Work out the finished part from the listing and answer in its coordinate system (mm). A direction names the side the tool comes from. Give positions to 0.01 mm unless a question says otherwise; leave off trailing zeros. Order: outer loops, then holes, each group sorted by start corner. A loop starts at its lowest first (then second) coordinate and runs counter-clockwise, first axis right, second up.
```python
from build123d import *

# Parameters (mm, degrees)
BOSS_EXTRUDE1_DEPTH = 10
SKETCH2_W           = 20
SKETCH2_H           = 14
BOSS_EXTRUDE2_DEPTH = 20
SKETCH3_W           = 20
SKETCH3_H           = 5
BOSS_EXTRUDE3_DEPTH = 20
SKETCH4_R           = 1.75
CUT_EXTRUDE1_DEPTH  = 84.402637848
CIRPATTERN1_COUNT   = 3
SKETCH5_R           = 2.5
CUT_EXTRUDE2_DEPTH  = 117.266161556
SKETCH8_W           = 20
SKETCH8_H           = 14
BOSS_EXTRUDE7_DEPTH = 5
SKETCH11_W          = 52
SKETCH11_H          = 52
BOSS_EXTRUDE8_DEPTH = 10
CUT_EXTRUDE3_DEPTH  = 7


with BuildPart() as part:
    # Sketch1 → Boss-Extrude1 (new body)
    with BuildSketch(Plane(origin=(0, 0, 0), x_dir=(1, 0, 0), z_dir=(0, 1, 0))):
        Polygon((0, 0), (-10, 5.773502692), (-10, 80), (10, 80), (10, 5.773502692), align=None)
    boss_extrude1 = extrude(amount=BOSS_EXTRUDE1_DEPTH)

    # Sketch2 → Boss-Extrude2 (add)
    with BuildSketch(Plane(origin=(0, 10, 0), x_dir=(1, 0, 0), z_dir=(0, 1, 0))):
        with Locations((0, 73)):
            Rectangle(SKETCH2_W, SKETCH2_H)
    boss_extrude2 = extrude(amount=BOSS_EXTRUDE2_DEPTH)

    # Sketch3 → Boss-Extrude3 (add)
    with BuildSketch(Plane(origin=(0, 30, 0), x_dir=(1, 0, 0), z_dir=(0, 1, 0))):
        with Locations((0, 77.5)):
            Rectangle(SKETCH3_W, SKETCH3_H)
        with Locations((0, 68.5)):
            Rectangle(SKETCH3_W, SKETCH3_H)
    boss_extrude3 = extrude(amount=BOSS_EXTRUDE3_DEPTH)

    # Sketch4 → Cut-Extrude1 (cut, symmetric)
    with BuildSketch(Plane.XY.offset(-66)):
        with Locations((0, 47)):
            Circle(SKETCH4_R)
    cut_extrude1 = extrude(amount=CUT_EXTRUDE1_DEPTH, both=True, mode=Mode.SUBTRACT)

    # CirPattern1: Boss-Extrude1, Boss-Extrude2, Boss-Extrude3, Cut-Extrude1 ×3 about axis
    cirpattern1_axis = Axis((0, 0, 0), (0, 1, 0))
    add([boss_extrude1.rotate(cirpattern1_axis, i * 360 / CIRPATTERN1_COUNT) for i in range(1, CIRPATTERN1_COUNT)])
    add([boss_extrude2.rotate(cirpattern1_axis, i * 360 / CIRPATTERN1_COUNT) for i in range(1, CIRPATTERN1_COUNT)])
    add([boss_extrude3.rotate(cirpattern1_axis, i * 360 / CIRPATTERN1_COUNT) for i in range(1, CIRPATTERN1_COUNT)])
    add([cut_extrude1.rotate(cirpattern1_axis, i * 360 / CIRPATTERN1_COUNT) for i in range(1, CIRPATTERN1_COUNT)], mode=Mode.SUBTRACT)

    # Sketch5 → Cut-Extrude2 (cut, through all)
    with BuildSketch(Plane(origin=(0, 10, 0), x_dir=(1, 0, 0), z_dir=(0, 1, 0))):
        with Locations(Location((0, 0, 0), (0, 0, 270))):
            Circle(SKETCH5_R)
    extrude(amount=-CUT_EXTRUDE2_DEPTH, mode=Mode.SUBTRACT)

    # Sketch8 → Boss-Extrude7 (add)
    with BuildSketch(Plane(origin=(0, 0, 0), x_dir=(1, 0, 0), z_dir=(0, 1, 0))):
        with Locations((0, 87)):
            Rectangle(SKETCH8_W, SKETCH8_H)
    extrude(amount=BOSS_EXTRUDE7_DEPTH)

    # Sketch11 → Boss-Extrude8 (add)
    with BuildSketch(Plane(origin=(0, 0, 0), x_dir=(1, 0, 0), z_dir=(0, 1, 0))):
        with Locations((0, 120)):
            Rectangle(SKETCH11_W, SKETCH11_H)
    extrude(amount=BOSS_EXTRUDE8_DEPTH)

    # Sketch12 → Cut-Extrude3 (cut)
    with BuildSketch(Plane(origin=(0, 10, 0), x_dir=(1, 0, 0), z_dir=(0, 1, 0))):
        Polygon((-21.1, 141.1), (-10.1, 141.1), (-10.1, 146), (10.1, 146), (10.1, 141.1), (21.1, 141.1), (21.1, 98.9), (-21.1, 98.9), align=None)
    extrude(amount=-CUT_EXTRUDE3_DEPTH, mode=Mode.SUBTRACT)


solid = part.part
```
1. Given P1, Ø3, axis at y = 2.5, z = -126, coming from the -X side; P2, Ø5.5, axis at x = 0, y = 47, coming from the +Z side; P3, Ø1.5, axis at y = 5, z = -30, coming from the -X side, each flat-ended and moving along its own axis, determine where each tip first touches the part or whether it passes through.
Findings below:
P1: stops at x = -26
P2: stops at z = -66
P3: stops at x = -10
2. The part is cut by section B-B (y = 16). Write down the section's boundary in (x, z), then the cut area to 3 significant figures.
Findings below:
outline: (-74.28, 31.34) - (-62.16, 24.34) - (-52.16, 41.66) - (-64.28, 48.66) - close; (-10, -80) - (10, -80) - (10, -66) - (-10, -66) - close; (52.16, 41.66) - (62.16, 24.34) - (74.28, 31.34) - (64.28, 48.66) - close
area: 840 mm2
3. Which of the six approach directions +Z, -Z, +X, -X, +Y, -Y give full straight-line access (tool end or side, diameter ignored) to faces 4 (the face through (-69.212, 24.65, 40.121)), 5 (the face through (-10.1, 7, -144)), 6 (the face through (-10, 8, -59)), 7 (the face through (63, 30, 36)), 8 (the face through (0, 30, -73))?
Findings below:
face 4: +Z, -X, +Y, -Y
face 5: -Z, +Y
face 6: -X, +Y, -Y
face 7: +Y
face 8: +X, -X, +Y
4. The mould has two halves that part along Z. Classify faces 1 (the face through (0, 40, -71)), 2 (the face through (0, 30, -66)), 3 (the face through (0, 50, -69)): pulls with the +Z half, pulls with the -Z half, needs draft (parallel to the pull), parting line crosses it, or undercut.
Findings below:
face 1: undercut
face 2: pulls with the +Z half
face 3: needs draft
5. The part is cut by section A-A (z = 0). Write down the section's boundary in (x, y), then the cut area to 3 significant figures.
Findings below:
outline: (-20, 0) - (-2.5, 0) - (-2.5, 10) - (-20, 10) - close; (2.5, 0) - (20, 0) - (20, 10) - (2.5, 10) - close
area: 350 mm2
6. Straight lines are drawn through the part: probe 1 along Y at (x, z) = (0, -69.6); probe 2 along Y at (x, z) = (-1.5, -93.5); probe 3 along X at (y, z) = (4, 0). For each, find the intervals that lie inside material, in ascending order.
Findings below:
probe 1: y = 0 to 45.25, 48.75 to 50
probe 2: y = 0 to 5
probe 3: x = -20 to -2.5, 2.5 to 20
7. The part is cut by section C-C (y = 35.5). Write down the section's boundary in (x, z), then the cut area to 3 significant figures.
Findings below:
outline: (-74.28, 31.34) - (-69.95, 28.84) - (-59.95, 46.16) - (-64.28, 48.66) - close; (-66.49, 26.84) - (-62.16, 24.34) - (-52.16, 41.66) - (-56.49, 44.16) - close; (-10, -80) - (10, -80) - (10, -75) - (-10, -75) - close; (-10, -71) - (10, -71) - (10, -66) - (-10, -66) - close; (52.16, 41.66) - (62.16, 24.34) - (66.49, 26.84) - (56.49, 44.16) - close; (59.95, 46.16) - (69.95, 28.84) - (74.28, 31.34) - (64.28, 48.66) - close
area: 600 mm2
8. The part is cut by section D-D (x = 16). Write down the section's boundary in (y, z).
Findings below:
outline: (0, -146) - (10, -146) - (10, -141.1) - (3, -141.1) - (3, -98.9) - (10, -98.9) - (10, -94) - (0, -94) - close; (0, -2.31) - (10, -2.31) - (10, 20.78) - (0, 20.78) - close
